from build123d import *

# Parameters (mm, degrees)
SKETCH1_W            = 29.2
SKETCH1_H            = 29.2
BOSS_EXTRUDE1_DEPTH  = 0.5
CUT_EXTRUDE1_START   = -2
CUT_EXTRUDE1_DEPTH   = 3
BOSS_EXTRUDE3_DEPTH  = 0.8
CUT_EXTRUDE4_START   = -1.5
CUT_EXTRUDE4_DEPTH   = 3.8
SKETCH10_OUTSIDE_W   = 53.166
SKETCH10_OUTSIDE_H   = 53.166
SKETCH10_OUTSIDE_W_2 = 26.2
SKETCH10_OUTSIDE_H_2 = 26.2
CUT_EXTRUDE9_DEPTH   = 0.8
CIRPATTERN1_COUNT    = 4
BOSS_EXTRUDE2_DEPTH  = 4.8
BOSS_EXTRUDE4_DEPTH  = 0.8
CUT_EXTRUDE10_DEPTH  = 0.1
BOSS_EXTRUDE5_DEPTH  = 5
FILLET1_R            = 0.5
SKETCH14_R           = 0.675
BOSS_EXTRUDE7_DEPTH  = 5


with BuildPart() as part:
    # Sketch1 → Boss-Extrude1 (new body, symmetric)
    with BuildSketch(Plane(origin=(0, 0, 0), x_dir=(1, 0, 0), z_dir=(0, 1, 0))):
        Rectangle(SKETCH1_W, SKETCH1_H)
    extrude(amount=BOSS_EXTRUDE1_DEPTH, both=True)

    # Sketch2 → Cut-Extrude1 (cut)
    with BuildSketch(Plane(origin=(0, 0.5, 0), x_dir=(1, 0, 0), z_dir=(0, 1, 0)).offset(CUT_EXTRUDE1_START)):
        with BuildLine():
            Line((-13.6, 4.75), (-13.6, -4.75))
            ThreePointArc((-13.6, -4.75), (-14.6, -5.75), (-15.6, -4.75))
            Line((-15.6, -4.75), (-15.6, 4.75))
            ThreePointArc((-15.6, 4.75), (-14.6, 5.75), (-13.6, 4.75))
        make_face()
    cut_extrude1 = extrude(amount=CUT_EXTRUDE1_DEPTH, mode=Mode.SUBTRACT)

    # Sketch6 → Boss-Extrude3 (add)
    with BuildSketch(Plane(origin=(0, 0.5, 0), x_dir=(1, 0, 0), z_dir=(0, 1, 0))):
        Polygon((19.940411229, 1.979898987), (-1.979898987, -19.940411229), (-19.940411229, -1.979898987), (1.979898987, 19.940411229), align=None)
    boss_extrude3 = extrude(amount=BOSS_EXTRUDE3_DEPTH)

    # Sketch4 → Cut-Extrude4 (cut)
    with BuildSketch(Plane(origin=(0, 0, 0), x_dir=(1, 0, 0), z_dir=(0, 1, 0)).offset(CUT_EXTRUDE4_START)):
        with BuildLine():
            Line((-14.22360169, 12.003810409), (-14.6, 12.655751406))
            Line((-14.6, 12.655751406), (-14.6, 14.6))
            Line((-14.6, 14.6), (-12.655751406, 14.6))
            Line((-12.655751406, 14.6), (-12.003810409, 14.22360169))
            ThreePointArc((-12.003810409, 14.22360169), (-11.66726189, 11.66726189), (-14.22360169, 12.003810409))
        make_face()
    cut_extrude4 = extrude(amount=CUT_EXTRUDE4_DEPTH, mode=Mode.SUBTRACT)

    # Sketch10 outside → Cut-Extrude9 (cut)
    with BuildSketch(Plane(origin=(0, 1.3, 0), x_dir=(1, 0, 0), z_dir=(0, 1, 0))):
        Rectangle(SKETCH10_OUTSIDE_W, SKETCH10_OUTSIDE_H)
        Rectangle(SKETCH10_OUTSIDE_W_2, SKETCH10_OUTSIDE_H_2, mode=Mode.SUBTRACT)
    cut_extrude9 = extrude(amount=-CUT_EXTRUDE9_DEPTH, mode=Mode.SUBTRACT)

    # CirPattern1: Cut-Extrude1, Cut-Extrude4 ×4 about axis
    cirpattern1_axis = Axis((0, 0, 0), (0, 1, 0))
    for i in range(1, CIRPATTERN1_COUNT):
        add(cut_extrude1.rotate(cirpattern1_axis, i * 360 / CIRPATTERN1_COUNT), mode=Mode.SUBTRACT)
        add(cut_extrude4.rotate(cirpattern1_axis, i * 360 / CIRPATTERN1_COUNT), mode=Mode.SUBTRACT)

    # Mirror3: Boss-Extrude3, Cut-Extrude9 across plane
    add(boss_extrude3.mirror(Plane.ZX))
    add(cut_extrude9.mirror(Plane.ZX), mode=Mode.SUBTRACT)

    # Sketch5 → Boss-Extrude2 (add)
    with BuildSketch(Plane.XZ.offset(0.5)):
        Polygon((4.772970773, 13.258252147), (8.732768748, 9.298454173), (11.030865787, 11.596551211), (7.071067812, 15.556349186), align=None)
        Polygon((9.298454173, 8.732768748), (13.258252147, 4.772970773), (15.556349186, 7.071067812), (11.596551211, 11.030865787), align=None)
    boss_extrude2 = extrude(amount=BOSS_EXTRUDE2_DEPTH)

    # Mirror1: Boss-Extrude2 across plane
    add(boss_extrude2.mirror(Plane(origin=(0, 0, 0), x_dir=(-0.707106781, 0, 0.707106781), z_dir=(0.707106781, 0, 0.707106781))))

    # Sketch11 → Boss-Extrude4 (add)
    with BuildSketch(Plane(origin=(0, 0.5, 0), x_dir=(1, 0, 0), z_dir=(0, 1, 0))):
        Polygon((-4.860512242, 13.1), (-9.527416998, 13.1), (-13.1, 9.527416998), (-13.1, 4.860512242), align=None)
    boss_extrude4 = extrude(amount=BOSS_EXTRUDE4_DEPTH)

    # Mirror4: Boss-Extrude4 across plane
    add(boss_extrude4.mirror(Plane(origin=(0, 0, 0), x_dir=(-0.707106781, 0, 0.707106781), z_dir=(0.707106781, 0, 0.707106781))))

    # Sketch12 → Cut-Extrude10 (cut)
    with BuildSketch(Plane(origin=(0, 1.3, 0), x_dir=(1, 0, 0), z_dir=(0, 1, 0))):
        Polygon((9.192388155, 9.192388155), (5.351397898, 7.601397898), (6.540737726, 7.601397898), (5.126524164, 6.187184335), (6.187184335, 5.126524164), (7.601397898, 6.540737726), (7.601397898, 5.351397898), align=None)
    extrude(amount=-CUT_EXTRUDE10_DEPTH, mode=Mode.SUBTRACT)

    # Sketch13 → Boss-Extrude5 (add)
    with BuildSketch(Plane.XZ.offset(0.5)):
        Polygon((-5.656854249, 10.960155108), (-10.960155108, 5.656854249), (-12.02081528, 6.717514421), (-11.844038585, 8.308504679), (-8.308504679, 11.844038585), (-6.717514421, 12.02081528), align=None)
    extrude(amount=BOSS_EXTRUDE5_DEPTH)

    # Fillet1
    fillet1_edges = [part.edges().sort_by_distance(p)[0] for p in [
        (-5.656854249, -3.4, 10.960155108),
        (-6.717514421, -3.4, 12.02081528),
        (-8.308504679, -3.4, 11.844038585),
        (-11.844038585, -3.4, 8.308504679),
        (-12.02081528, -3.4, 6.717514421),
        (-10.960155108, -3.4, 5.656854249),
    ]]
    fillet(fillet1_edges, radius=FILLET1_R)

    # Sketch14 → Boss-Extrude7 (add)
    with BuildSketch(Plane.XZ.offset(0.5)):
        with Locations((-12.6, 2.6)):
            Circle(SKETCH14_R)
        with Locations((-12.6, 4.6)):
            Circle(SKETCH14_R)
    extrude(amount=BOSS_EXTRUDE7_DEPTH)


solid = part.part
Can you work these out from the model? Positions are in its coordinate system, mm. A direction names the side the tool comes from. Coordinates: 2 decimals unless noted, no trailing zeros. Order: outer loops, then holes, each group sorted by start corner. A loop starts at its lowest first (then second) coordinate and runs counter-clockwise, first axis right, second up. Notation, with made-up numbers: M 67.5,82.5 L 88.5,82.5 A19 ccw 88.5,98.5 Z; hole C 11,39 d7. An arc over 180 degrees is marked long. Write item = value, one per line.
(1) Suppose I cut it at C-C on z = 2.6. Please give me the cut outline in (x, y) (3 decimals), plus the area to 3 significant figures.
Results are:
outline = M -13.6,-0.5 L -13.275,-0.5 L -13.275,-5.5 L -11.925,-5.5 L -11.925,-1.3 L 13.1,-1.3 L 13.1,-0.5 L 13.6,-0.5 L 13.6,0.5 L 13.1,0.5 L 13.1,1.3 L -13.1,1.3 L -13.1,0.5 L -13.6,0.5 Z
area = 74.9 mm2
(2) For faces 4 (the face through (-5.465, -0.007, 13.901)), 5 (the face through (-9.023, -2.866, -13.604)), 6 (the face through (-10.93, -0.89, 10.99)), which set-ups out of +Z, -Z, +X, -X, +Y, -Y let a thin tool reach every point of the face, with its end or its side?
Results are:
face_4 = +Z, +Y, -Y
face_5 = -Z, -X, -Y
face_6 = +Z, -X, -Y
(3) I need wall thicknesses on line 1 along X through (y, z) = (0.25, -8); line 2 along Y through (x, z) = (4, -8); line 3 along Z through (x, y) = (2.5, -1). Which ranges of each line are inside material? Lowest first, please. Write a range as [from, to].
Results are:
line_1 = [-14.6, 14.6]
line_2 = [-1.3, 1.3]
line_3 = [-13.1, 13.1]
(4) Suppose I cut it at A-A on y = -2. State how many separate pieces and enclosed holes the cut face has, plus the area to 3 significant figures.
Results are:
separate_pieces = 7
enclosed_holes = 0
area = 93.0 mm2
(5) If we mould it in two halves opening along X, with no side actions, what happens to faces 1 (the face through (9, 0, -14.6)), 2 (the face through (-13.6, 0, 0)), 3 (the face through (-11.638, -0.007, -11.697))? For each: pulls with the +X half, pulls with the -X half, needs draft (parallel to the pull), parting line crosses it, or undercut.
Results are:
face_1 = needs draft
face_2 = pulls with the -X half
face_3 = undercut
(6) For pin 1 Ø1.5 at (y, z) = (-3, 11.5) entering from -X; pin 2 Ø3 at (x, z) = (-6, -10.5) entering from -Y; pin 3 Ø1.5 at (x, y) = (6, 0) entering from +Z, each with a flat end and sliding along its axis, tell me the tip position at first contact or that it passes through.
Results are:
pin_1 = -9.4
pin_2 = -5.3
pin_3 = 15.04
(7) Suppose I cut it at B-B on x = 0.5. Please give me the cut outline in (y, z).
Results are:
outline = M -1.3,-13.1 L -0.5,-13.1 L -0.5,-13.6 L 0.5,-13.6 L 0.5,-13.1 L 1.3,-13.1 L 1.3,13.1 L 0.5,13.1 L 0.5,13.6 L -0.5,13.6 L -0.5,13.1 L -1.3,13.1 Z
